Can you work these out from the model? Positions are in its coordinate system, mm. Face numbers are marked on the shaded views. A direction names the side the tool comes from. Give positions to 0.01 mm unless a question says otherwise; leave off trailing zeros. Loops run counter-clockwise (first coordinate to the right, second up) from the corner with the lowest first, then second, coordinate; pieces in that order, holes last. Notation, with made-up numbers: M 35.25,56.25 L 58.25,56.25 A16 ccw 58.25,81.25 Z; hole C -33,-33 d3. An arc over 180 degrees is marked long. Use CSV: the item, a comma, the result in double quotes.
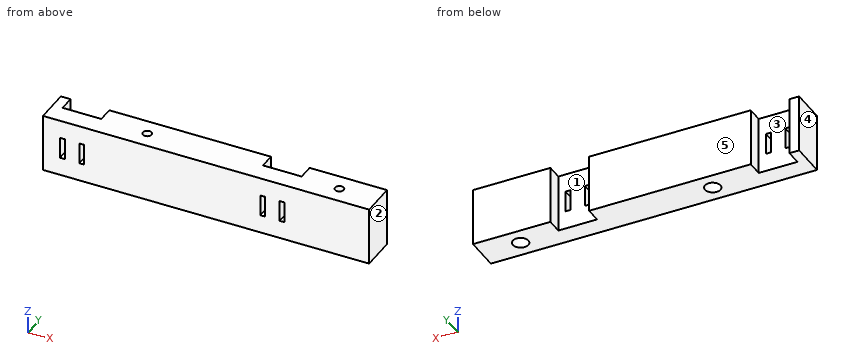
Autodesk Inventor part; units mm, degrees
ref_plane "작업 평면1" through (18, 12.5444, -60) normal (0, 0, -1) x (-1, 0, 0)
ref_plane "YZ Plane" through (0, 0, 0) normal (1, 0, 0) x (0, 1, 0)
ref_plane "XZ Plane" through (0, 0, 0) normal (0, 1, 0) x (-1, 0, 0)
ref_plane "작업 평면1" through (18, 12.5444, -60) normal (0, 0, -1) x (-1, 0, 0)
sketch "스케치1" plane through (18, 12.5444, -60) normal (0, 0, -1) x (-1, 0, 0)
  circle A0 centre (149.27, -9) radius 2.25
  circle A1 centre (50, -9) radius 2.25
  line L0 (60.4781, -35) -> (62.5565, -31.4)
  line L1 (62.5565, -31.4) -> (66.7134, -31.4)
  line L2 (66.7134, -31.4) -> (68.7919, -35)
  line L3 (68.7919, -35) -> (66.7134, -38.6)
  line L4 (66.7134, -38.6) -> (62.5565, -38.6)
  line L5 (62.5565, -38.6) -> (60.4781, -35)
  line L6 (161.8265, -38.6) -> (159.748, -35)
  line L7 (159.748, -35) -> (161.8265, -31.4)
  line L8 (161.8265, -31.4) -> (165.9834, -31.4)
  line L9 (165.9834, -31.4) -> (168.0619, -35)
  line L10 (168.0619, -35) -> (165.9834, -38.6)
  line L11 (165.9834, -38.6) -> (161.8265, -38.6)
  line L12 (30, -50) -> (198.5399, -50)
  line L13 (198.5399, -50) -> (198.5399, 0)
  line L14 (0, 0) -> (198.5399, 0)
  line L15 (0, 0) -> (0, -12.5444)
  line L16 (0, -12.5444) -> (30, -12.5444)
  line L17 (30, -12.5444) -> (30, -50)
  line L18 (30, 0) -> (30, -18)
  line L19 (30, -18) -> (198.5399, -18)
  line L20 (198.5399, -18) -> (198.5399, 0)
  line L21 (176.0399, 8) -> (191.0399, 8)
  line L22 (72.5, 8) -> (87.5, 8)
  line L23 (193.5399, -8) -> (173.5399, -8)
  line L24 (173.5399, -8) -> (173.5399, 0)
  line L25 (193.5399, 0) -> (193.5399, -8)
  line L26 (90, -8) -> (70, -8)
  line L27 (70, -8) -> (70, 0)
  line L28 (90, 0) -> (90, -8)
  line L29 (70, 0) -> (30, 0)
  line L30 (198.5399, 0) -> (193.5399, 0)
  line L31 (173.5399, 0) -> (90, 0)
  point P0 (18, -12.5444)
  point P1 (80, -8)
  point P2 (80, 8)
  point P3 (183.5399, -8)
  point P4 (183.5399, 8)
  point P5 (70, 0)
  dimension "d1" = 18
  dimension "d6" = 8
  dimension "d7" = 8
extrude "돌출1" add sketch "스케치1" along normal blind 30 contours L17 L18 L14 L27 L26 L28 L24 L23 L25 L13 L19
sketch "스케치2" plane through (18, 12.5444, -90) normal (0, 0, -1) x (-1, 0, 0)
  circle A0 centre (149.27, -9) radius 2.25
  circle A1 centre (50, -9) radius 2.25
  circle A2 centre (149.27, -9) radius 4
  circle A3 centre (50, -9) radius 4
  point P0 (18, -12.5444)
  dimension "d10" = 8
  dimension "d11" = 8
extrude "돌출2" cut sketch "스케치2" against normal blind 25 contours A0 | A1 | A2 | A3
sketch "스케치3" plane through (-175.5399, 4.5444, -60) normal (0, 1, 0) x (1, 0, 0)
  line L0 (0, 0) -> (20, 0)
  line L1 (20, 0) -> (20, 30)
  line L2 (0, 30) -> (20, 30)
  line L3 (0, 0) -> (0, 30)
  line L4 (103.5399, 0) -> (123.5399, 0)
  line L5 (123.5399, 0) -> (123.5399, 30)
  line L6 (103.5399, 30) -> (123.5399, 30)
  line L7 (103.5399, 0) -> (103.5399, 30)
  line L8 (5, 20.5) -> (15, 20.5)
  line L9 (15, 20.5) -> (15, 9.5)
  line L10 (15, 9.5) -> (5, 9.5)
  line L11 (5, 9.5) -> (5, 20.5)
  line L12 (5, 20.5) -> (15, 9.5) construction
  line L13 (15, 20.5) -> (5, 9.5) construction
  line L14 (108.5399, 20.5) -> (118.5399, 20.5)
  line L15 (118.5399, 20.5) -> (118.5399, 9.5)
  line L16 (118.5399, 9.5) -> (108.5399, 9.5)
  line L17 (108.5399, 9.5) -> (108.5399, 20.5)
  line L18 (108.5399, 20.5) -> (118.5399, 9.5) construction
  line L19 (118.5399, 20.5) -> (108.5399, 9.5) construction
  line L20 (3.75, 20.5) -> (6.25, 20.5)
  line L21 (6.25, 20.5) -> (6.25, 9.5)
  line L22 (6.25, 9.5) -> (3.75, 9.5)
  line L23 (3.75, 9.5) -> (3.75, 20.5)
  line L24 (3.75, 20.5) -> (6.25, 9.5) construction
  line L25 (6.25, 20.5) -> (3.75, 9.5) construction
  line L26 (13.75, 20.5) -> (16.25, 20.5)
  line L27 (16.25, 20.5) -> (16.25, 9.5)
  line L28 (16.25, 9.5) -> (13.75, 9.5)
  line L29 (13.75, 9.5) -> (13.75, 20.5)
  line L30 (13.75, 20.5) -> (16.25, 9.5) construction
  line L31 (16.25, 20.5) -> (13.75, 9.5) construction
  line L32 (107.2899, 20.5) -> (109.7899, 20.5)
  line L33 (109.7899, 20.5) -> (109.7899, 9.5)
  line L34 (109.7899, 9.5) -> (107.2899, 9.5)
  line L35 (107.2899, 9.5) -> (107.2899, 20.5)
  line L36 (107.2899, 20.5) -> (109.7899, 9.5) construction
  line L37 (109.7899, 20.5) -> (107.2899, 9.5) construction
  line L38 (117.2899, 20.5) -> (119.7899, 20.5)
  line L39 (119.7899, 20.5) -> (119.7899, 9.5)
  line L40 (119.7899, 9.5) -> (117.2899, 9.5)
  line L41 (117.2899, 9.5) -> (117.2899, 20.5)
  line L42 (117.2899, 20.5) -> (119.7899, 9.5) construction
  line L43 (119.7899, 20.5) -> (117.2899, 9.5) construction
  point P0 (175.5399, -60)
  point P1 (10, 15)
  point P2 (113.5399, 15)
  point P3 (5, 15)
  point P4 (15, 15)
  point P5 (108.5399, 15)
  point P6 (118.5399, 15)
  point P7 (118.5399, 20.5)
  point P8 (117.2899, 20.5)
  point P9 (117.2899, 9.5)
  point P10 (118.5399, 9.5)
  point P11 (108.5399, 9.5)
  point P12 (109.7899, 20.5)
  point P13 (108.5399, 20.5)
  point P14 (13.75, 20.5)
  point P15 (13.75, 9.5)
  point P16 (15, 9.5)
  point P17 (15, 20.5)
  point P18 (6.25, 20.5)
  point P19 (5, 20.5)
  point P20 (5, 9.5)
  dimension "d14" = 10
  dimension "d15" = 11
  dimension "d16" = 10
  dimension "d17" = 11
  dimension "d18" = 2.5
  dimension "d19" = 2.5
  dimension "d20" = 2.5
  dimension "d21" = 2.5
extrude "돌출3" cut sketch "스케치3" against normal through all contours L8 L21 L10 L11 | L11 L22 L23 L20 | L8 L9 L10 L29 | L26 L27 L28 L9 | L14 L33 L16 L17 | L17 L34 L35 L32 | L14 L15 L16 L41 | L38 L39 L40 L15
properties part number "side_ToF_mount"
Q1. For the marked faces 1 and 2, which set-ups out of +Z, -Z, +X, -X, +Y, -Y let a thin tool reach every point of the face, with its end or its side?
Model answer:
face 1,"+Z, -Z, +Y"
face 2,"+Z, -Z, +X, +Y, -Y"
Q2. I want a section at C-C, the plane z = -74.75. State how many separate pieces and enclosed holes the cut face has, then the cut area to 3 significant figures.
Model answer:
separate pieces,"5"
enclosed holes,"2"
area,"2,510 mm2"
Q3. I want a section at A-A, the plane x = -32. Please give me the cut outline in (y, z), then the cut area to 4 significant figures.
Model answer:
outline,"M -5.46,-90 L -0.46,-90 L -0.46,-65 L 1.29,-65 L 1.29,-60 L -5.46,-60 Z; M 5.79,-65 L 7.54,-65 L 7.54,-90 L 12.54,-90 L 12.54,-60 L 5.79,-60 Z"
area,"317.5 mm2"
Q4. Please list where these lines run through material, in increasing order: L1, parallel to Y at x = -131.27, z = -62.5; L2, parallel to X at y = 11.75, z = -75.75; L3, parallel to Y at x = -131.27, z = -76.75. Write a range as from..to.
Model answer:
L1,"-5.46..1.29, 5.79..12.54"
L2,"-180.54..-175.54, -155.54..-72, -52..-12"
L3,"-5.46..-0.46, 7.54..12.54"
Q5. If we mould it in two halves opening along X, with no side actions, what happens to the marked faces 3, 4 and 5? For each: released by +X, released by -X, zero draft, split by the parting line, or undercut.
Model answer:
face 3,"undercut"
face 4,"released by -X"
face 5,"zero draft"
Q6. I want a section at B-B, the plane y = 9. Please give me the cut outline in (x, z).
Model answer:
outline,"M -180.54,-90 L -175.54,-90 L -175.54,-60 L -180.54,-60 Z; M -155.54,-90 L -72,-90 L -72,-60 L -155.54,-60 Z; M -52,-90 L -12,-90 L -12,-60 L -52,-60 Z"
Q7. I want a section at D-D, the plane y = -3. Please give me the cut outline in (x, z).
Model answer:
outline,"M -180.54,-90 L -12,-90 L -12,-60 L -180.54,-60 Z; hole M -171.79,-80.5 L -169.29,-80.5 L -169.29,-69.5 L -171.79,-69.5 Z; hole M -161.79,-80.5 L -159.29,-80.5 L -159.29,-69.5 L -161.79,-69.5 Z; hole M -68.25,-80.5 L -65.75,-80.5 L -65.75,-69.5 L -68.25,-69.5 Z; hole M -58.25,-80.5 L -55.75,-80.5 L -55.75,-69.5 L -58.25,-69.5 Z"
